```python
from build123d import *

# Parameters (mm, degrees)
SKETCH1_R           = 1.7
SKETCH1_W           = 40.64
SKETCH1_H           = 40.64
SKETCH1_W_2         = 6.441435375
SKETCH1_H_2         = 11.864636979
BOSS_EXTRUDE1_DEPTH = 3.175


with BuildPart() as part:
    # Sketch1 → Boss-Extrude1 (new body)
    with BuildSketch(Plane(origin=(0, 0, 0), x_dir=(1, 0, 0), z_dir=(0, 1, 0))):
        Polygon((-89.999999959, 100.000000025), (-82.146123441, 100.000000025), (-82.146123441, 87.012397876), (-54.188171851, 87.012397876), (-54.188171851, 100.000000025), (-41.018658576, 100.000000025), (-41.018658576, 88.447791729), (-23.524827511, 88.447791729), (-23.524827511, 100.000000025), (43.67960641, 100.000000025), (43.67960641, 87.012397876), (61.636212859, 87.012397876), (61.636212859, 100.000000025), (89.999999959, 100.000000025), (89.999999959, 45.570881719), (38.364340903, 45.570881719), (38.364340903, 20.032473827), (89.999999959, 20.032473827), (89.999999959, -100.000000025), (21.816000041, -100.000000025), (21.816000041, -90.000000025), (-1.805999959, -90.000000025), (-1.805999959, -100.000000025), (-20.869596106, -100.000000025), (-20.869596106, -70.58952404), (-82.146123441, -70.58952404), (-82.146123441, -100.000000025), (-89.999999959, -100.000000025), align=None)
        with Locations(Location((-86.499999959, 96.111111133, 0), (0, 0, 270))):
            Circle(SKETCH1_R, mode=Mode.SUBTRACT)
        with Locations(Location((-4.999999959, 96.500000025, 0), (0, 0, 270))):
            Circle(SKETCH1_R, mode=Mode.SUBTRACT)
        with Locations(Location((86.500000041, 96.111111224, 0), (0, 0, 270))):
            Circle(SKETCH1_R, mode=Mode.SUBTRACT)
        with Locations(Location((-86.499999959, -96.111111133, 0), (0, 0, 270))):
            Circle(SKETCH1_R, mode=Mode.SUBTRACT)
        with Locations(Location((-6.989999959, -95.000000025, 0), (0, 0, 270))):
            Circle(SKETCH1_R, mode=Mode.SUBTRACT)
        with Locations(Location((27.000000041, -95.000000025, 0), (0, 0, 270))):
            Circle(SKETCH1_R, mode=Mode.SUBTRACT)
        with Locations(Location((86.500000041, -96.111111224, 0), (0, 0, 270))):
            Circle(SKETCH1_R, mode=Mode.SUBTRACT)
        with Locations(Location((86.499999959, 15.999999975, 0), (0, 0, 270))):
            Circle(SKETCH1_R, mode=Mode.SUBTRACT)
        with Locations(Location((-86.499999959, -30.000000025, 0), (0, 0, 270))):
            Circle(SKETCH1_R, mode=Mode.SUBTRACT)
        with Locations((-37.475629524, 39.402171336)):
            Rectangle(SKETCH1_W, SKETCH1_H, mode=Mode.SUBTRACT)
        with Locations((23.20161852, -82.635134039)):
            Rectangle(SKETCH1_W_2, SKETCH1_H_2, mode=Mode.SUBTRACT)
    extrude(amount=BOSS_EXTRUDE1_DEPTH)


solid = part.part
```
For this review, take the finished solid that the model builds, in its own axes (mm). Coordinates: 2 decimals unless noted, no trailing zeros. Order: outer loops, then holes, each group sorted by start corner. A loop starts at its lowest first (then second) coordinate and runs counter-clockwise, first axis right, second up. Notation, with made-up numbers: (-39.5, -16) -> (-26.5, -16) arc R18 cw to (-26.5, 15) -> close; hole circle Ø11 at (-40, -36). An arc over 180 degrees is marked (long way). Use CSV: the item, a comma, the result in double quotes. Start each with the question number.
Item 1: Insertion check: pin 1 (1 mm diameter, centred on x = -33.5, y = 1, fed in from +Z). The pin has a flat end and moves straight along its axis. Give the tip position at first contact, or say it passes through.
Item 2: Wall thickness on probe 1 along Z at (x, y) = (46, 1.5); probe 2 along Z at (x, y) = (-43, 2.25); probe 3 along X at (y, z) = (1.45, 30): over which ranges is each line inside the solid? List them lowest first.
Item 3: We need section A-A, the plane x = -30. Give the boundary of the cut face in (y, z) (3 decimals).
Item 4: We need section B-B, the plane y = 2.1. Give the number of separate pieces and of enclosed holes in the cut face, then the cut area to 3 significant figures.
Item 5: We need section C-C, the plane x = -70.5. Give the boundary of the cut face in (y, z) (3 decimals), then the cut area to 3 significant figures.
Derived:
1,pin 1,"stops at z = 70.59"
2,probe 1,"z = -87.01 to -45.57, -20.03 to 100"
2,probe 2,"z = -100 to -59.72, -19.08 to 70.59"
2,probe 3,"x = -90 to -88.2, -84.8 to 90"
3,outline,"(0, -88.448) -> (3.175, -88.448) -> (3.175, -59.722) -> (0, -59.722) -> close; (0, -19.082) -> (3.175, -19.082) -> (3.175, 70.59) -> (0, 70.59) -> close"
4,separate pieces,"1"
4,enclosed holes,"11"
4,area,"30,000 mm^2"
5,outline,"(0, -87.012) -> (3.175, -87.012) -> (3.175, 70.59) -> (0, 70.59) -> close"
5,area,"500 mm^2"
